Geometry check sheet. Reference: the model listing, model coordinates, mm. A direction names the side the tool comes from. Give positions to 0.01 mm unless a question says otherwise; leave off trailing zeros. Order: outer loops, then holes, each group sorted by start corner. A loop starts at its lowest first (then second) coordinate and runs counter-clockwise, first axis right, second up.
from build123d import *

# Parameters (mm, degrees)
BOSS_EXTRUDE1_DEPTH     = 5
CUT_EXTRUDE1_DEPTH      = 1
CUT_EXTRUDE1_DEPTH_BACK = 6


with BuildPart() as part:
    # Sketch3 → Boss-Extrude1 (new body)
    with BuildSketch(Plane.XY.offset(-218.000000001)):
        Polygon((-282.039404117, 408.696835159), (-340.287524909, 408.696835159), (-352.932442284, 416.294668041), (-352.932442284, 427.528407952), (-313.380404337, 427.528407952), align=None)
    extrude(amount=-BOSS_EXTRUDE1_DEPTH)

    # Sketch4 → Cut-Extrude1 (cut, two sides)
    with BuildSketch(Plane(origin=(0, 0, -223.000000001), x_dir=(-1, 0, 0), z_dir=(0, 0, -1))) as cut_extrude1_sk:
        Polygon((318.275750374, 408.696835159), (314.075750374, 408.696835159), (314.075750374, 412.696835159), (312.075750374, 412.696835159), (312.075750374, 415.496835159), (314.075750374, 415.496835159), (314.075750374, 425.496835159), (318.275750374, 425.496835159), (318.275750374, 415.496835159), (320.275750374, 415.496835159), (320.275750374, 412.696835159), (318.275750374, 412.696835159), align=None)
        Polygon((338.843972624, 412.696835159), (340.843972624, 412.696835159), (340.843972624, 415.496835159), (338.843972624, 415.496835159), (338.843972624, 425.496835159), (334.643972624, 425.496835159), (334.643972624, 415.496835159), (332.643972624, 415.496835159), (332.643972624, 412.696835159), (334.643972624, 412.696835159), (334.643972624, 408.696835159), (338.843972624, 408.696835159), align=None)
    extrude(amount=CUT_EXTRUDE1_DEPTH, mode=Mode.SUBTRACT)
    extrude(cut_extrude1_sk.sketch, amount=-CUT_EXTRUDE1_DEPTH_BACK, mode=Mode.SUBTRACT)


solid = part.part
Item 1: Sectioned sample at C-C (y = 420.5). Enter the section's corners in (x, z), and give its area (3 significant figures).
Reported:
outline: (-352.93, -223) - (-338.84, -223) - (-338.84, -218) - (-352.93, -218) - close; (-334.64, -223) - (-318.28, -223) - (-318.28, -218) - (-334.64, -218) - close; (-314.08, -223) - (-301.68, -223) - (-301.68, -218) - (-314.08, -218) - close
area: 214 mm2
Item 2: Gauge pin test, flat ends, axial feed: pin 1 (1 mm diameter, centred on x = -299.5, z = -219, fed in from +Y); pin 2 (0.8 mm diameter, centred on y = 414.5, z = -221.5, fed in from +X); pin 3 (2 mm diameter, centred on y = 411.5, z = -220, fed in from +X); pin 4 (1 mm diameter, centred on x = -340.5, z = -220.5, fed in from -Y). Record the tip position at first contact, or that the pin passes through.
Reported:
pin 1: stops at y = 419.49
pin 2: stops at x = -291.03
pin 3: stops at x = -285.04
pin 4: stops at y = 408.7
Item 3: Draft check along Y on faces 4 (the flat face through (-319, 412.697, -221)), 5 (the flat face through (-316, 425.497, -221)), 6 (the flat face through (-314.076, 420, -221)). Enter one of: released by +Y, released by -Y, zero draft, split by the parting line, or undercut.
Reported:
face 4: undercut
face 5: released by -Y
face 6: zero draft
Item 4: Set-up check for faces 1 (the flat face through (-318.276, 411, -221)), 2 (the flat face through (-340, 408.697, -220)), 3 (the flat face through (-334, 412.697, -221)): record each of +Z, -Z, +X, -X, +Y, -Y from which the full face is reachable in a straight line by a thin tool's end or side.
Reported:
face 1: +Z, -Z, -Y
face 2: +Z, -Z, +X, -X, -Y
face 3: +Z, -Z
Item 5: Scan lines: L1, parallel to X at y = 412.75, z = -218.75 (3 decimals); L2, parallel to X at y = 417.25, z = -219.65; L3, parallel to Y at x = -338, z = -221.55. Record each from-to range of solid material in increasing order.
Reported:
L1: x = -347.033 to -340.844, -332.644 to -320.276, -312.076 to -288.785
L2: x = -352.93 to -338.84, -334.64 to -318.28, -314.08 to -296.27
L3: y = 425.5 to 427.53
Item 6: Sectioned sample at A-A (y = 424). Enter the section's corners in (x, z).
Reported:
outline: (-352.93, -223) - (-338.84, -223) - (-338.84, -218) - (-352.93, -218) - close; (-334.64, -223) - (-318.28, -223) - (-318.28, -218) - (-334.64, -218) - close; (-314.08, -223) - (-307.51, -223) - (-307.51, -218) - (-314.08, -218) - close
Item 7: Sectioned sample at D-D (x = -306.5). Enter the section's corners in (y, z).
Reported:
outline: (408.7, -223) - (423.39, -223) - (423.39, -218) - (408.7, -218) - close
